```python
from build123d import *

# Parameters (mm, degrees)
SKETCH1_W           = 300
SKETCH1_H           = 100
BOSS_EXTRUDE1_DEPTH = 5
SKETCH7_R           = 10
BOSS_EXTRUDE5_DEPTH = 25
SKETCH10_R          = 4
BOSS_EXTRUDE6_DEPTH = 50
LPATTERN1_COUNT     = 3
LPATTERN1_PITCH     = 100


with BuildPart() as part:
    # Sketch1 → Boss-Extrude1 (new body)
    with BuildSketch(Plane(origin=(0, 0, 0), x_dir=(1, 0, 0), z_dir=(0, 1, 0))):
        Rectangle(SKETCH1_W, SKETCH1_H)
    extrude(amount=BOSS_EXTRUDE1_DEPTH)

    # Sketch7 → Boss-Extrude5 (add)
    with BuildSketch(Plane(origin=(150, 0, 0), x_dir=(0, 0, -1), z_dir=(1, 0, 0))):
        with Locations((50.954154719, 10.172311349)):
            Circle(SKETCH7_R)
    boss_extrude5 = extrude(amount=-BOSS_EXTRUDE5_DEPTH)

    # Sketch10 → Boss-Extrude6 (add)
    with BuildSketch(Plane(origin=(150, 0, 0), x_dir=(0, 0, -1), z_dir=(1, 0, 0))):
        with Locations((50.954154719, 10.172311349)):
            Circle(SKETCH10_R)
    boss_extrude6 = extrude(amount=-BOSS_EXTRUDE6_DEPTH)

    # LPattern1: Boss-Extrude5, Boss-Extrude6 ×3
    with Locations(*[Vector(-0.999994942, 0, 0.0031805) * (i * LPATTERN1_PITCH) for i in range(1, LPATTERN1_COUNT)]):
        add(boss_extrude5)
        add(boss_extrude6)


solid = part.part
```
Input: part model. Units: mm. Frame: model coordinates. A direction names the side the tool comes from. Coordinates: 2 decimals unless noted, no trailing zeros. Loops run counter-clockwise (first coordinate to the right, second up) from the corner with the lowest first, then second, coordinate; pieces in that order, holes last.
Q1. Section D-D, the plane x = 43.5. Return the cut outline in (y, z), and give its area (3 significant figures).
Results are:
outline: (0, -50) - (0.19, -50) arc R10 ccw (long way) to (5, -42.08) - (5, 50) - (0, 50) - close
area: 788 mm2
Q2. Section C-C, the plane x = -108. Return the cut outline in (y, z).
Results are:
outline: (0, -50) - (5, -50) - (5, 50) - (0, 50) - close
Q3. Mould query, pull axis X, two halves, no side actions, for faces 1 (the flat face through (-150, 2, 1)), 2 (the flat face through (-2, 2, 50)), 3 (the flat face through (-2, 2, -50)). Classes: +X half, -X half, draft (parallel to the pull), parting line (faces both ways), or undercut.
Results are:
face 1: -X half
face 2: draft
face 3: undercut
Q4. Set-up query: faces 4 (the flat face through (100, 10, -51)), 5 (the flat face through (150, 4, -18)), 6 (the cylindrical face through (-87.324, 7.738, -47.144)), 7 (the flat face through (25.001, 10, -55)). Return all of +Z, -Z, +X, -X, +Y, -Y with unobstructed straight access to the full face (end or side cutting, diameter ignored); none if empty.
Results are:
face 4: +Z, -Z, +Y
face 5: +Z, -Z, +X, +Y, -Y
face 6: -X
face 7: none
Q5. Section B-B, the plane z = 30.5. Return the cut outline in (x, y).
Results are:
outline: (-150, 0) - (150, 0) - (150, 5) - (-150, 5) - close
Q6. Contact query for flat-ended pins moving along their axis: pin 1 (2 mm diameter, centred on x = -70, y = 7.5, fed in from +Z); pin 2 (1.5 mm diameter, centred on x = -65.5, y = 2.5, fed in from -Z); pin 3 (10 mm diameter, centred on x = -8, z = 1, fed in from +Y). Output: stop coordinate, or through.
Results are:
pin 1: stops at z = -40.46
pin 2: stops at z = -57.53
pin 3: stops at y = 5
Q7. Line query: line 1 along X through (y, z) = (16, -51.5); line 2 along Z through (x, y) = (9, 8.5); line 3 along Y through (x, z) = (27, -24). Output: solid intervals per line, ascending.
Results are:
line 1: x = -75 to -50, 25 to 50, 125 to 150
line 2: z = -54.27 to -47
line 3: y = 0 to 5
Q8. Section A-A, the plane x = 107. Return the cut outline in (y, z), and give its area (3 significant figures).
Results are:
outline: (0, -50) - (5, -50) - (5, 50) - (0, 50) - close; circle Ø8 at (10.17, -50.95)
area: 550 mm2
